Autodesk Inventor part; units mm, degrees
ref_plane "YZ Plane" through (0, 0, 0) normal (1, 0, 0) x (0, 1, 0)
ref_plane "XZ Plane" through (0, 0, 0) normal (0, 1, 0) x (-1, 0, 0)
ref_plane "XY Plane" through (0, 0, 0) normal (0, 0, 1) x (1, 0, 0)
sketch "Sketch1" plane through (0, 0, 0) normal (0, 0, 1) x (1, 0, 0)
  line L0 (2.6197, -0.0625) -> (1.364, -2.2375)
  line L1 (1.2557, -2.3) -> (-1.2557, -2.3)
  line L2 (-1.364, -2.2375) -> (-2.6197, -0.0625)
  line L3 (-2.6197, 0.0625) -> (-1.364, 2.2375)
  line L4 (-1.2557, 2.3) -> (1.2557, 2.3)
  line L5 (1.364, 2.2375) -> (2.6197, 0.0625)
  arc A0 (-1.2557, 2.3) -> (-1.364, 2.2375) centre (-1.2557, 2.175) ccw
  arc A1 (-2.6197, 0.0625) -> (-2.6197, -0.0625) centre (-2.5115, 0) ccw
  arc A2 (-1.364, -2.2375) -> (-1.2557, -2.3) centre (-1.2557, -2.175) ccw
  arc A3 (1.2557, -2.3) -> (1.364, -2.2375) centre (1.2557, -2.175) ccw
  arc A4 (2.6197, -0.0625) -> (2.6197, 0.0625) centre (2.5115, 0) ccw
  arc A5 (1.364, 2.2375) -> (1.2557, 2.3) centre (1.2557, 2.175) ccw
  point P0 (0, 0)
  point P1 (2.6558, 0)
  point P2 (1.3279, -2.3)
  point P3 (-1.3279, -2.3)
  point P4 (-2.6558, 0)
  point P5 (-1.3279, 2.3)
  point P6 (1.3279, 2.3)
  dimension "d36" = 4.6
  dimension "d37" = 0.125
extrude "Extrusion1" add sketch "Sketch1" along normal blind 6
sketch "草圖5" plane through (0, 0, 6) normal (0, 0, 1) x (1, 0, 0)
  point P0 (0, 0)
  point P1 (0, 0)
hole "孔2" at (0, 0, 6) direction (0, 0, -1) diameter 2.459 end through all
chamfer "倒角2" distance 0.125 angle 45 2 edges at (0, 1.2295, 6) (0, 1.2295, 0)
sketch "草圖6" plane through (0, 0, 0) normal (0, 1, 0) x (-1, 0, 0)
  line L0 (-2.3, 0) -> (-2.8, 0)
  line L1 (-2.8, 6) -> (-2.3, 6)
  line L2 (-2.8, 6) -> (-2.8, 5.7)
  line L3 (-2.8, 0) -> (-2.8, 0.3)
  arc A0 (-2.3, 6) -> (-2.8, 5.7) centre (-2.3, 5.4333) ccw
  arc A1 (-2.8, 0.3) -> (-2.3, 0) centre (-2.3, 0.5667) ccw
  line L4 (0, 0) -> (0, 6)
  dimension "d48" = 6
  dimension "d50" = 2.3
  dimension "d51" = 2.3
  dimension "d52" = 0.5
  dimension "d53" = 0.3
  dimension "d54" = 0.3
revolve "迴轉2" cut sketch "草圖6" angle 360 about axis through (0, 0, 0) along (0, 0, 1)
properties part number "nut_rod_M3_8"
Work out the finished part from the listing and answer in its coordinate system (mm). Coordinates: 2 decimals unless noted, no trailing zeros. Loops run counter-clockwise (first coordinate to the right, second up) from the corner with the lowest first, then second, coordinate; pieces in that order, holes last. Notation, with made-up numbers: (70, 63.25) -> (112, 63.25) arc R6 ccw to (112, 74.25) -> close; hole circle Ø4 at (-15, -18.75). An arc over 180 degrees is marked (long way). Write each question's results on one line, items separated by ' | '. Start each with the question number.
1) The mould has two halves that part along Y. Classify faces 1 (the cylindrical face through (0.748, 0.976, 2.96)), 2 (the flat face through (2.001, -1.135, 2.958)), 3 (the flat face through (0, 2.3, 3)): pulls with the +Y half, pulls with the -Y half, needs draft (parallel to the pull), parting line crosses it, or undercut.
2) Find section A-A on z = 5.25. Determine the outline of the cut face in (x, y), then the cut area to 3 significant figures.
3) Consider line 1 along Y through (x, z) = (0, 4); line 2 along X through (y, z) = (0, 2.9); line 3 along Y through (x, z) = (-0.5, 1). Determine where each line is inside the solid, lowest interval first.
4) A flat-ended cylindrical pin translates along its axis: P1, Ø1, axis at y = 1, z = 3.5, coming from the +X side. Find the tip coordinate at first contact, or state that the pin passes through.
Response values:
1) face 1: undercut | face 2: pulls with the -Y half | face 3: pulls with the +Y half
2) outline: (-2.62, -0.06) -> (-1.36, -2.24) arc R0.12 ccw to (-1.26, -2.3) -> (1.26, -2.3) arc R0.13 ccw to (1.36, -2.24) -> (2.62, -0.06) arc R0.12 ccw to (2.62, 0.06) -> (1.36, 2.24) arc R0.12 ccw to (1.26, 2.3) -> (-1.26, 2.3) arc R0.13 ccw to (-1.36, 2.24) -> (-2.62, 0.06) arc R0.12 ccw to start; hole circle Ø2.46 at (0, 0) | area: 13.6 mm^2
3) line 1: y = -2.3 to -1.23, 1.23 to 2.3 | line 2: x = -2.64 to -1.23, 1.23 to 2.64 | line 3: y = -2.3 to -1.12, 1.12 to 2.3
4) P1: stops at x = 2.37
